from build123d import *

# Parameters (mm, degrees)
F2_R          = 1.459965
F3_DEPTH      = 23.4188
F3_DEPTH_BACK = 25.4
F5_R          = 6.151073
F5_R_2        = 6.494421
F5_R_3        = 6.5989
F5_R_4        = 6.538752
F6_DEPTH      = 38.608
F6_DEPTH_BACK = 35.814


with BuildPart() as f1:
    # F0 (on Right) → F1 (revolve)
    with BuildSketch(Plane.YZ):
        with BuildLine():
            Line((-3, 20), (-3, 0))
            Line((-3, 0), (3, 0))
            Line((3, 0), (3, 20.092177))
            Line((3, 20.092177), (2, 20.092177))
            ThreePointArc((2, 20.092177), (0.038764, 18.363927), (-2, 20))
            Line((-2, 20), (-3, 20))
        make_face()
    revolve(axis=Axis((0, 0, 0), (0, 1, 0)))


with BuildPart() as f3:
    # F2 (on Front) → F3 (new body, two sides)
    with BuildSketch(Plane.XZ) as f3_sk:
        Circle(F2_R)
    extrude(amount=F3_DEPTH)
    extrude(f3_sk.sketch, amount=-F3_DEPTH_BACK)


with BuildPart() as f1_1:
    add(f1.part)

    # F4: cut F3
    add(f3.part, mode=Mode.SUBTRACT)


with BuildPart() as f6:
    # F5 (on Front) → F6 (new body, two sides)
    with BuildSketch(Plane.XZ) as f6_sk:
        with Locations((0, 11.43)):
            Circle(F5_R)
        with Locations((-10.139517, 0)):
            Circle(F5_R_2)
        with Locations((0, -11.06129)):
            Circle(F5_R_3)
        with Locations((11.614354, 0)):
            Circle(F5_R_4)
    extrude(amount=F6_DEPTH)
    extrude(f6_sk.sketch, amount=-F6_DEPTH_BACK)


with BuildPart() as f1_2:
    add(f1_1.part)

    # F7: cut F6
    add(f6.part, mode=Mode.SUBTRACT)


solid = f1_2.part
Here's how the part is built. I have some questions about the finished solid (model axes, mm). Round coordinates to 2 decimals unless told otherwise and drop trailing zeros. Write each loop counter-clockwise with the first axis right and the second up, starting at its lowest first coordinate (ties: lowest second). Pieces come first, ordered by that corner, then holes. Notation, with made-up numbers: (-24, -25.5) -> (-15, -25.5) arc R15 cw to (-15, 3.5) -> close; hole circle Ø9 at (84, 47). An arc over 180 degrees is marked (long way). One line per item, written item: value.
1) Suppose I cut it at A-A on x = 0. List the corners of the cut face in (y, z) for me.
Filled sheet:
outline: (-3, -20) -> (-2, -20) arc R2.03 cw to (2, -20.09) -> (3, -20.09) -> (3, -17.66) -> (-3, -17.66) -> close; (-3, -4.46) -> (3, -4.46) -> (3, -1.46) -> (-3, -1.46) -> close; (-3, 1.46) -> (3, 1.46) -> (3, 5.28) -> (-3, 5.28) -> close; (-3, 17.58) -> (3, 17.58) -> (3, 20.09) -> (2, 20.09) arc R2.03 cw to (-2, 20) -> (-3, 20) -> close
2) Suppose I cut it at B-B on z = 0. List the corners of the cut face in (x, y) for me.
Filled sheet:
outline: (-20.09, 2) arc R2.03 cw to (-20, -2) -> (-20, -3) -> (-16.63, -3) -> (-16.63, 3) -> (-20.09, 3) -> close; (-3.65, -3) -> (-1.46, -3) -> (-1.46, 3) -> (-3.65, 3) -> close; (1.46, -3) -> (5.08, -3) -> (5.08, 3) -> (1.46, 3) -> close; (18.15, -3) -> (20, -3) -> (20, -2) arc R2.03 cw to (20.09, 2) -> (20.09, 3) -> (18.15, 3) -> close
3) If I drill on line 1 (X direction, y = 0.9, z = 4.5); line 2 (X direction, y = 0.9, z = -2.5); line 3 (X direction, y = -1, z = -5.5), over which ranges is the centre line in solid material (lowest first)? Write a range as [from, to].
Filled sheet:
line 1: x = [-18.02, -14.82], [-5.46, 6.87], [16.36, 18.02]
line 2: x = [-18.41, -16.13], [-4.15, 5.57], [17.66, 18.41]
line 3: x = [-17.79, -13.59], [-6.69, -3.55], [3.55, 8.08], [15.15, 17.79]
4) Suppose I cut it at C-C on y = 0.4. List the corners of the cut face in (x, z) for me.
Filled sheet:
outline: circle Ø36.81 at (0, 0); hole circle Ø12.99 at (-10.14, 0); hole circle Ø13.2 at (0, -11.06); hole circle Ø12.3 at (0, 11.43); hole circle Ø2.92 at (0, 0); hole circle Ø13.08 at (11.61, 0)
5) I'm going to push a flat-ended pin straight in: pin 1 Ø2 at (y, z) = (1.5, 12.5) entering from -X. Where does the tip first touch, or does it pass through?
Filled sheet:
pin 1: stops at x = -16.38
6) We'd pull the mould along Z, two halves only. Please class faces 1 (the face through (17.654, -0.042, -2.504)), 2 (the face through (-0.8, -0.04, 17.53)), 3 (the face through (-19.524, -2.507, -4.336)), 4 (the face through (0, -3, 4)): released by +Z, released by -Z, zero draft, split by the parting line, or undercut.
Filled sheet:
face 1: undercut
face 2: undercut
face 3: split by the parting line
face 4: zero draft
7) Suppose I cut it at D-D on x = 4.5. Give the number of separate pieces and of enclosed holes in the cut face, plus the area to 3 significant figures.
Filled sheet:
separate pieces: 3
enclosed holes: 0
area: 116 mm2
